```python
from build123d import *

# Parameters (mm, degrees)
BOX008_W               = 6.5
BOX008_H               = 20
BOX008_DEPTH           = 10.5
BOX007_W               = 6.5
BOX007_H               = 20
BOX007_DEPTH           = 10.5
BOX009_W               = 6.5
BOX009_H               = 20
BOX009_DEPTH           = 10.5
BOX010_W               = 6.5
BOX010_H               = 20
BOX010_DEPTH           = 10.5
BOX011_W               = 6.5
BOX011_H               = 20
BOX011_DEPTH           = 10.5
BOX013_W               = 6.5
BOX013_H               = 20
BOX013_DEPTH           = 10.5
BOX012_W               = 6.5
BOX012_H               = 20
BOX012_DEPTH           = 10.5
BOX006_W               = 6.5
BOX006_H               = 20
BOX006_DEPTH           = 10.5
SKETCH008_W            = 28
SKETCH008_H            = 33
EXTRUDE001_DEPTH       = 4.5
SKETCH007_R            = 13
SKETCH007_R_2          = 1.65
EXTRUDE_DEPTH          = 40
BOX002_W               = 133.36
BOX002_H               = 150
BOX002_DEPTH           = 16
FILLET002_R            = 7
BOX003_W               = 154
BOX003_H               = 140
BOX003_DEPTH           = 26
SKETCH004_R            = 51.75
PAD003_DEPTH           = 6
PAD004_DEPTH           = 35
SKETCH006_R            = 2.35
PAD005_DEPTH           = 35
PAD_DEPTH              = 7.9
SKETCH002_R            = 59
PAD001_DEPTH           = 25
SKETCH003_R            = 2.85
PAD002_DEPTH           = 34
BOX_W                  = 184
BOX_H                  = 200
BOX_DEPTH              = 305
FILLET_R               = 20
BOX001_W               = 204
BOX001_H               = 225
BOX001_DEPTH           = 325
FILLET001_R            = 30
BOX004_W               = 141
BOX004_H               = 132
BOX004_DEPTH           = 10
BOX004_PLACEMENT_ANGLE = 45
BOX005_W               = 184
BOX005_H               = 203
BOX005_DEPTH           = 10


with BuildPart() as cubo006:
    # Box008 → Box008 (new body)
    with BuildSketch(Plane(origin=(-52.5, 0, 60), x_dir=(1, 0, 0), z_dir=(0, 0, 1))):
        with Locations((3.25, 10)):
            Rectangle(BOX008_W, BOX008_H)
    extrude(amount=BOX008_DEPTH)


with BuildPart() as cubo005:
    # Box007 → Box007 (new body)
    with BuildSketch(Plane(origin=(46, 0, 158), x_dir=(1, 0, 0), z_dir=(0, 0, 1))):
        with Locations((3.25, 10)):
            Rectangle(BOX007_W, BOX007_H)
    extrude(amount=BOX007_DEPTH)


with BuildPart() as cubo007:
    # Box009 → Box009 (new body)
    with BuildSketch(Plane(origin=(-52.5, 0, 158), x_dir=(1, 0, 0), z_dir=(0, 0, 1))):
        with Locations((3.25, 10)):
            Rectangle(BOX009_W, BOX009_H)
    extrude(amount=BOX009_DEPTH)


with BuildPart() as cubo008:
    # Box010 → Box010 (new body)
    with BuildSketch(Plane(origin=(28.5, 0, 198), x_dir=(1, 0, 0), z_dir=(0, 0, 1))):
        with Locations((3.25, 10)):
            Rectangle(BOX010_W, BOX010_H)
    extrude(amount=BOX010_DEPTH)


with BuildPart() as cubo009:
    # Box011 → Box011 (new body)
    with BuildSketch(Plane(origin=(28.5, 0, 262), x_dir=(1, 0, 0), z_dir=(0, 0, 1))):
        with Locations((3.25, 10)):
            Rectangle(BOX011_W, BOX011_H)
    extrude(amount=BOX011_DEPTH)


with BuildPart() as cubo011:
    # Box013 → Box013 (new body)
    with BuildSketch(Plane(origin=(-35, 0, 198), x_dir=(1, 0, 0), z_dir=(0, 0, 1))):
        with Locations((3.25, 10)):
            Rectangle(BOX013_W, BOX013_H)
    extrude(amount=BOX013_DEPTH)


with BuildPart() as cubo010:
    # Box012 → Box012 (new body)
    with BuildSketch(Plane(origin=(-35, 0, 262), x_dir=(1, 0, 0), z_dir=(0, 0, 1))):
        with Locations((3.25, 10)):
            Rectangle(BOX012_W, BOX012_H)
    extrude(amount=BOX012_DEPTH)


with BuildPart() as obj1:
    # Box006 → Box006 (new body)
    with BuildSketch(Plane(origin=(46, 0, 60), x_dir=(1, 0, 0), z_dir=(0, 0, 1))):
        with Locations((3.25, 10)):
            Rectangle(BOX006_W, BOX006_H)
    extrude(amount=BOX006_DEPTH)

    # Fusion003: union Cubo006, Cubo005, Cubo007, Cubo008, Cubo009, Cubo011, Cubo010
    add(cubo006.part)
    add(cubo005.part)
    add(cubo007.part)
    add(cubo008.part)
    add(cubo009.part)
    add(cubo011.part)
    add(cubo010.part)


with BuildPart() as obj1_1:
    # Fusion003 placement: moved
    add(obj1.part.moved(Location((0, 12, 0))))


with BuildPart() as extrude001:
    # Sketch008 → Extrude001 (new body)
    with BuildSketch(Plane.XZ):
        with Locations((0, 120)):
            Rectangle(SKETCH008_W, SKETCH008_H)
    extrude(amount=EXTRUDE001_DEPTH)


with BuildPart() as extrude001_1:
    # Extrude001 placement: moved
    add(extrude001.part.moved(Location((0, 220, 0))))


with BuildPart() as conector:
    # Sketch007 → Extrude (new body)
    with BuildSketch(Plane.XZ):
        with Locations((0, 120)):
            Circle(SKETCH007_R)
        with Locations((9.5, 132)):
            Circle(SKETCH007_R_2)
        with Locations((-9.5, 108)):
            Circle(SKETCH007_R_2)
    extrude(amount=EXTRUDE_DEPTH)


with BuildPart() as conector_1:
    # Extrude placement: moved
    add(conector.part.moved(Location((0, 226, 0))))

    # Fusion: union Extrude001
    add(extrude001_1.part)


with BuildPart() as conector_2:
    # Fusion placement: moved
    add(conector_1.part.moved(Location((0, 5, 0))))


with BuildPart() as fusion002:
    # Box002 → Box002 (new body)
    with BuildSketch(Plane(origin=(-66.68, 0, 10), x_dir=(1, 0, 0), z_dir=(0, 0, 1))):
        with Locations((66.68, 75)):
            Rectangle(BOX002_W, BOX002_H)
    extrude(amount=BOX002_DEPTH)

    # Fillet002
    fillet002_edges = [fusion002.edges().sort_by_distance(p)[0] for p in [
        (-66.68, 75, 26),
        (-66.68, 75, 10),
        (66.68, 75, 26),
        (66.68, 75, 10),
    ]]
    fillet(fillet002_edges, radius=FILLET002_R)

    # Fusion002: union Conector
    add(conector_2.part)


with BuildPart() as puerto:
    # Box003 → Box003 (new body)
    with BuildSketch(Plane(origin=(-77, 10, 10), x_dir=(1, 0, 0), z_dir=(0, 0, 1))):
        with Locations((77, 70)):
            Rectangle(BOX003_W, BOX003_H)
    extrude(amount=BOX003_DEPTH)


with BuildPart() as obj2:
    # Sketch004 → Pad003 (new body)
    with BuildSketch(Plane.XZ):
        with Locations((0, 235)):
            Circle(SKETCH004_R)
    extrude(amount=-PAD003_DEPTH)

    # Sketch005 → Pad004 (join)
    with BuildSketch(Plane.XZ):
        with BuildLine():
            Line((-38.729833, 225), (-44, 225))
            Line((-44, 225), (-44, 245))
            Line((-44, 245), (-38.729833, 245))
            ThreePointArc((38.729833, 245), (0, 275), (-38.729833, 245))
            Line((38.729833, 245), (44, 245))
            Line((44, 245), (44, 225))
            Line((44, 225), (38.729833, 225))
            ThreePointArc((-38.729833, 225), (0, 195), (38.729833, 225))
        make_face()
    extrude(amount=-PAD004_DEPTH)

    # Sketch006 → Pad005 (join)
    with BuildSketch(Plane.XZ):
        with Locations((-31.82, 266.819221)):
            Circle(SKETCH006_R)
        with Locations((31.82, 266.819221)):
            Circle(SKETCH006_R)
        with Locations((31.82, 203.18)):
            Circle(SKETCH006_R)
        with Locations((-31.82, 203.18)):
            Circle(SKETCH006_R)
    extrude(amount=-PAD005_DEPTH)


with BuildPart() as obj3:
    # Sketch → Pad (new body)
    with BuildSketch(Plane.XZ):
        with BuildLine():
            Line((-37.019041, 181.175), (37.019041, 181.175))
            ThreePointArc((67.175, 151.019041), (54.23509, 168.23509), (37.019041, 181.175))
            Line((67.175, 151.019041), (67.175, 76.980959))
            ThreePointArc((37.019041, 46.825), (54.23509, 59.76491), (67.175, 76.980959))
            Line((37.019041, 46.825), (-37.019041, 46.825))
            ThreePointArc((-67.175, 76.980959), (-54.23509, 59.76491), (-37.019041, 46.825))
            Line((-67.175, 76.980959), (-67.175, 151.019041))
            ThreePointArc((-37.019041, 181.175), (-54.23509, 168.23509), (-67.175, 151.019041))
        make_face()
    extrude(amount=-PAD_DEPTH)

    # Sketch002 → Pad001 (join)
    with BuildSketch(Plane.XZ):
        with Locations((0, 114)):
            Circle(SKETCH002_R)
    extrude(amount=-PAD001_DEPTH)

    # Sketch003 → Pad002 (join)
    with BuildSketch(Plane.XZ):
        with Locations((-49.0732, 163.07)):
            Circle(SKETCH003_R)
        with Locations((49.0732, 163.07)):
            Circle(SKETCH003_R)
        with Locations((49.0732, 64.93)):
            Circle(SKETCH003_R)
        with Locations((-49.0732, 64.93)):
            Circle(SKETCH003_R)
    extrude(amount=-PAD002_DEPTH)


with BuildPart() as obj4:
    # Box → Box (new body)
    with BuildSketch(Plane(origin=(-92, 15, 10), x_dir=(1, 0, 0), z_dir=(0, 0, 1))):
        with Locations((92, 100)):
            Rectangle(BOX_W, BOX_H)
    extrude(amount=BOX_DEPTH)

    # Fillet
    fillet_edges = [obj4.edges().sort_by_distance(p)[0] for p in [
        (-92, 15, 162.5),
        (-92, 115, 315),
        (-92, 215, 162.5),
        (92, 15, 162.5),
        (92, 115, 315),
        (92, 215, 162.5),
        (0, 15, 315),
        (0, 215, 315),
    ]]
    fillet(fillet_edges, radius=FILLET_R)


with BuildPart() as cut002:
    # Box001 → Box001 (new body)
    with BuildSketch(Plane(origin=(-102, 0, 0), x_dir=(1, 0, 0), z_dir=(0, 0, 1))):
        with Locations((102, 112.5)):
            Rectangle(BOX001_W, BOX001_H)
    extrude(amount=BOX001_DEPTH)

    # Fillet001
    fillet001_edges = [cut002.edges().sort_by_distance(p)[0] for p in [
        (-102, 0, 162.5),
        (-102, 112.5, 325),
        (-102, 225, 162.5),
        (102, 0, 162.5),
        (102, 112.5, 325),
        (102, 225, 162.5),
        (0, 0, 325),
        (0, 225, 325),
    ]]
    fillet(fillet001_edges, radius=FILLET001_R)

    # Cut: cut obj4
    add(obj4.part, mode=Mode.SUBTRACT)

    # Cut001: cut obj3
    add(obj3.part, mode=Mode.SUBTRACT)

    # Cut002: cut obj2
    add(obj2.part, mode=Mode.SUBTRACT)


with BuildPart() as cubo002:
    # Box004 → Box004 (new body)
    with BuildSketch(Plane.XY):
        with Locations((70.5, 66)):
            Rectangle(BOX004_W, BOX004_H)
    extrude(amount=BOX004_DEPTH)


with BuildPart() as cubo002_1:
    # Box004 placement: moved
    add(cubo002.part.moved(Location((-95, 120, 0))).rotate(Axis((-95, 120, 0), (0, 0, -1)), BOX004_PLACEMENT_ANGLE))


with BuildPart() as cut005:
    # Box005 → Box005 (new body)
    with BuildSketch(Plane(origin=(-92, 13, 0), x_dir=(1, 0, 0), z_dir=(0, 0, 1))):
        with Locations((92, 101.5)):
            Rectangle(BOX005_W, BOX005_H)
    extrude(amount=BOX005_DEPTH)

    # Cut003: cut Cubo002
    add(cubo002_1.part, mode=Mode.SUBTRACT)


with BuildPart() as cut005_1:
    # Cut003 placement: moved
    add(cut005.part.moved(Location((0, 0, 181))))

    # Fusion001: union Puerto, Cut002
    add(puerto.part)
    add(cut002.part)

    # Cut004: cut Fusion002
    add(fusion002.part, mode=Mode.SUBTRACT)

    # Cut005: cut obj1
    add(obj1_1.part, mode=Mode.SUBTRACT)


solid = cut005_1.part
```
For this review, take the finished solid that the model builds, in its own axes (mm). A direction names the side the tool comes from. Coordinates: 2 decimals unless noted, no trailing zeros. Order: outer loops, then holes, each group sorted by start corner. A loop starts at its lowest first (then second) coordinate and runs counter-clockwise, first axis right, second up. Notation, with made-up numbers: (34, -27.5) -> (62, -27.5) arc R24 ccw to (62, -1.5) -> close; hole circle Ø4 at (-28, -22). An arc over 180 degrees is marked (long way). Use CSV: the item, a comma, the result in double quotes. Start each with the question number.
Item 1: Wall thickness on probe 1 along Z at (x, y) = (6, 98.5); probe 2 along X at (y, z) = (56, 32); probe 3 along X at (y, z) = (161.5, 291.5): over which ranges is each line inside the solid? List them lowest first.
Item 2: We need section C-C, the plane z = 235. Give the boundary of the cut face in (x, y), then the cut area to 3 significant figures.
Item 3: For faces 5 (the face through (-102, 111, 145)), 6 (the face through (54.02, 3.89, 59.55)), 7 (the face through (-86.297, 21.014, 243.728)), list the 3-axis set-ups (+Z, -Z, +X, -X, +Y, -Y) from which the entire face can be reached by the end or side of a thin tool; tool diameter is ignored.
Item 4: Insertion check: pin 1 (4 mm diameter, centred on x = -42.5, y = 9.5, fed in from +Z); pin 2 (1.6 mm diameter, centred on x = 40.5, y = 11, fed in from +Z); pin 3 (6.5 mm diameter, centred on y = 2.5, z = 96.5, fed in from -X). Each pin has a flat end and moves straight along its axis. Give the tip position at first contact, or say it passes through.
Item 5: Draft analysis for pull direction Z (two halves, no side actions). For faces 1 (the face through (61, 7.9, 115)), 2 (the face through (92.979, 8.555, 149.565)), 3 (the face through (-1, 215, 242)), 4 (the face through (1.008, 8.555, 315.979)), state which applies: pulls with the +Z half, pulls with the -Z half, needs draft (parallel to the pull), parting line crosses it, or undercut.
Item 6: We need section B-B, the plane y = 145. Give the number of separate pieces and of enclosed holes in the cut face, then the cut area to 3 significant figures.
Derived:
1,probe 1,"z = 0 to 10, 26 to 36, 315 to 325"
1,probe 2,"x = -102 to -92, -77 to 77, 92 to 102"
1,probe 3,"x = -102 to -92, 92 to 102"
2,outline,"(-102, 30) arc R30 ccw to (-72, 0) -> (-51.75, 0) -> (-51.75, 6) -> (-44, 6) -> (-44, 15) -> (-72, 15) arc R20 cw to (-92, 35) -> (-92, 195) arc R20 cw to (-72, 215) -> (72, 215) arc R20 cw to (92, 195) -> (92, 35) arc R20 cw to (72, 15) -> (44, 15) -> (44, 6) -> (51.75, 6) -> (51.75, 0) -> (72, 0) arc R30 ccw to (102, 30) -> (102, 195) arc R30 ccw to (72, 225) -> (-72, 225) arc R30 ccw to (-102, 195) -> close"
2,area,"7,260 mm^2"
3,face 5,"+Z, -Z, -X, +Y, -Y"
3,face 6,"-Y"
3,face 7,"none"
4,pin 1,"stops at z = 318.62"
4,pin 2,"stops at z = 318.85"
4,pin 3,"stops at x = -89.66"
5,face 1,"undercut"
5,face 2,"needs draft"
5,face 3,"undercut"
5,face 4,"pulls with the +Z half"
6,separate pieces,"1"
6,enclosed holes,"2"
6,area,"12,400 mm^2"
